Design review of the part built by this model. Coordinates are the model's own, in mm. Face numbers are marked on the shaded views. A direction names the side the tool comes from. Coordinates: 2 decimals unless noted, no trailing zeros. Write each loop counter-clockwise with the first axis right and the second up, starting at its lowest first coordinate (ties: lowest second). Pieces come first, ordered by that corner, then holes. Notation, with made-up numbers: (43.5, 5.25) -> (90.5, 5.25) arc R3 cw to (90.5, 9.25) -> close; hole circle Ø10 at (55, 34). An arc over 180 degrees is marked (long way). One line per question, with ' | ' between items. Start each with the question number.
Q1. For P1, Ø20, axis at x = 23.5, y = -28.5, coming from the +Z side; P2, Ø6, axis at x = -22.5, y = -57.5, coming from the -Z side; P3, Ø1.5, axis at x = 49.5, z = 1, coming from the -Y side, all flat-tipped, find the tip position at first contact; note any pin that passes through.
Q2. Wall thickness on probe 1 along X at (y, z) = (-21, -30); probe 2 along Y at (x, z) = (24, -9); probe 3 along Z at (x, y) = (88, -28): over which ranges is each line inside the solid? List them lowest first.
Q3. Add section B-B on z = 44. State the section outline as (x, y) points.
Q4. Add section C-C on x = 92.5. State the section outline as (y, z) points, and give its area (3 significant figures).
Q5. Add section D-D on y = -57. State the section outline as (x, z) points, and give its area (3 significant figures).
Q6. Add section A-A on y = -40. State the section outline as (x, z) points, and give its area (3 significant figures).
Q7. For the marked faces 1 and 2, list the 3-axis set-ups (+Z, -Z, +X, -X, +Y, -Y) from which the entire face can be reached by the end or side of a thin tool; tool diameter is ignored.
Q8. Draft analysis for pull direction Y (two halves, no side actions). For the marked faces 3, 4, 5 and 6, state which applies: pulls with the +Y half, pulls with the -Y half, needs draft (parallel to the pull), parting line crosses it, or undercut.
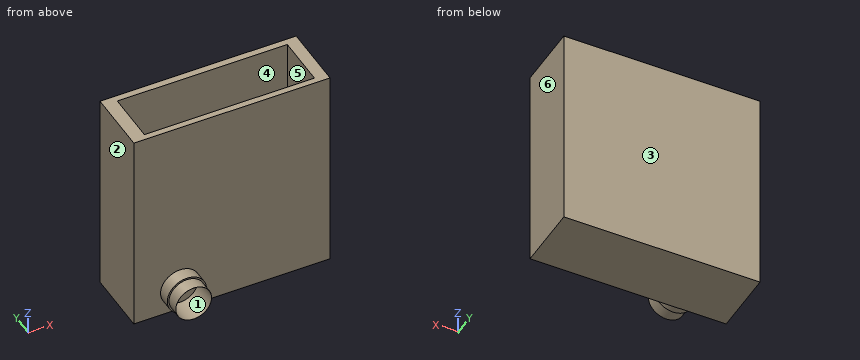
from build123d import *

# Parameters (mm, degrees)
F0_W     = 150
F0_H     = 160
F1_DEPTH = 50
F2_W     = 130
F2_H     = 40
F3_DEPTH = 155
F4_R     = 15
F5_DEPTH = 10
F6_R     = 13.698165
F7_DEPTH = 10
F8_R     = 13.6531
F9_DEPTH = 20


with BuildPart() as f1:
    # F0 (on Front) → F1 (new body)
    with BuildSketch(Plane.XZ):
        with Locations((28.931955, -3.273388)):
            Rectangle(F0_W, F0_H)
    extrude(amount=F1_DEPTH)

    # F2 (on face) → F3 (cut)
    with BuildSketch(Plane.XY.offset(76.726612)):
        with Locations((29.457796, -25.269221)):
            Rectangle(F2_W, F2_H)
    extrude(amount=-F3_DEPTH, mode=Mode.SUBTRACT)

    # F4 (on face) → F5 (join)
    with BuildSketch(Plane.XZ.offset(50)):
        with Locations((-10.681064, -63.932007)):
            Circle(F4_R)
    extrude(amount=F5_DEPTH)

    # F6 (on face) → F7 (join)
    with BuildSketch(Plane.XZ.offset(60)):
        with Locations((-10.681064, -63.932007)):
            Circle(F6_R)
    extrude(amount=F7_DEPTH)

    # F8 (on face) → F9 (cut)
    with BuildSketch(Plane.XZ.offset(70)):
        with Locations((-10.681064, -63.932007)):
            Circle(F8_R)
    extrude(amount=-F9_DEPTH, mode=Mode.SUBTRACT)


solid = f1.part
Output values:
1) P1: stops at z = -78.27 | P2: stops at z = -76.07 | P3: stops at y = -50
2) probe 1: x = -46.07 to -35.54, 94.46 to 103.93 | probe 2: y = -50 to -45.27, -5.27 to 0 | probe 3: z = -83.27 to -78.27
3) outline: (-46.07, -50) -> (103.93, -50) -> (103.93, 0) -> (-46.07, 0) -> close; hole (-35.54, -45.27) -> (94.46, -45.27) -> (94.46, -5.27) -> (-35.54, -5.27) -> close
4) outline: (-50, -83.27) -> (0, -83.27) -> (0, 76.73) -> (-5.27, 76.73) -> (-5.27, -78.27) -> (-45.27, -78.27) -> (-45.27, 76.73) -> (-50, 76.73) -> close | area: 1,800 mm2
5) outline: circle Ø30 at (-10.68, -63.93); hole circle Ø27.31 at (-10.68, -63.93) | area: 121 mm2
6) outline: (-46.07, -83.27) -> (103.93, -83.27) -> (103.93, 76.73) -> (94.46, 76.73) -> (94.46, -78.27) -> (-35.54, -78.27) -> (-35.54, 76.73) -> (-46.07, 76.73) -> close | area: 3,850 mm2
7) face 1: -Y | face 2: +Z, -Z, -X, +Y, -Y
8) face 3: pulls with the +Y half | face 4: undercut | face 5: undercut | face 6: needs draft
